from build123d import *

# Parameters (mm, degrees)
EXTRUDE001_DEPTH = 3
EXTRUDE_DEPTH    = 3
SKETCH_W         = 60
SKETCH_H         = 7
SKETCH_R         = 1.4
PAD_DEPTH        = 10
SKETCH001_W      = 60
SKETCH001_H      = 5
PAD001_DEPTH     = 3.5
SKETCH002_W      = 14
SKETCH002_H      = 5
PAD002_DEPTH     = 12
SKETCH003_R      = 1.9
PAD003_DEPTH     = 4


with BuildPart() as m2_5_pocket:
    # Polygon001 → Extrude001 (new body)
    with BuildSketch(Plane(origin=(56.6, 3, 10), x_dir=(1, 0, 0), z_dir=(0, 0, -1))):
        Polygon((1.45, 2.511474), (2.9, 0), (1.45, -2.511474), (-1.45, -2.511474), (-2.9, 0), (-1.45, 2.511474), align=None)
    extrude(amount=EXTRUDE001_DEPTH)


with BuildPart() as m2_5_pocket001:
    # Polygon → Extrude (new body)
    with BuildSketch(Plane(origin=(3.1, 3, 10), x_dir=(1, 0, 0), z_dir=(0, 0, -1))):
        Polygon((1.45, 2.511474), (2.9, 0), (1.45, -2.511474), (-1.45, -2.511474), (-2.9, 0), (-1.45, 2.511474), align=None)
    extrude(amount=EXTRUDE_DEPTH)


with BuildPart() as cut001:
    # Sketch → Pad (new body)
    with BuildSketch(Plane.XY):
        with Locations((30, 3.5)):
            Rectangle(SKETCH_W, SKETCH_H)
        with Locations((3.1, 3)):
            Circle(SKETCH_R, mode=Mode.SUBTRACT)
        with Locations((56.6, 3)):
            Circle(SKETCH_R, mode=Mode.SUBTRACT)
    extrude(amount=PAD_DEPTH)

    # Sketch001 → Pad001 (new body)
    with BuildSketch(Plane(origin=(0, 7, 0), x_dir=(-1, 0, 0), z_dir=(0, 1, 0))):
        with Locations((-30, 7.5)):
            Rectangle(SKETCH001_W, SKETCH001_H)
    extrude(amount=PAD001_DEPTH)

    # Sketch002 → Pad002 (new body)
    with BuildSketch(Plane(origin=(0, 7, 0), x_dir=(-1, 0, 0), z_dir=(0, 1, 0))):
        with Locations((-7, 7.5)):
            Rectangle(SKETCH002_W, SKETCH002_H)
    extrude(amount=PAD002_DEPTH)

    # Sketch003 → Pad003 (new body)
    with BuildSketch(Plane(origin=(0, 0, 5), x_dir=(1, 0, 0), z_dir=(0, 0, -1))):
        with Locations((7.3, -14.5)):
            Circle(SKETCH003_R)
    extrude(amount=PAD003_DEPTH)

    # Cut: cut M2.5 pocket001
    add(m2_5_pocket001.part, mode=Mode.SUBTRACT)

    # Cut001: cut M2.5 pocket
    add(m2_5_pocket.part, mode=Mode.SUBTRACT)


solid = cut001.part
Verification items for the finished model (mm, model axes). A direction names the side the tool comes from. Round coordinates to 2 decimals unless told otherwise and drop trailing zeros. Write each loop counter-clockwise with the first axis right and the second up, starting at its lowest first coordinate (ties: lowest second). Pieces come first, ordered by that corner, then holes.
(1) Depth check by flat-ended pin: pin 1 Ø2 at (y, z) = (13, 4.5) entering from +X; pin 2 Ø10 at (x, y) = (8, 12.5) entering from -Z; pin 3 Ø5.5 at (x, z) = (37.5, 8) entering from +Y; pin 4 Ø1.5 at (x, y) = (56.5, 2.5) entering from +Z. Enter the tip coordinate at first touch or a pass-through.
Returned:
pin 1: stops at x = 14
pin 2: stops at z = 1
pin 3: stops at y = 10.5
pin 4: passes through
(2) Section check C-C (z = 6.25). Enter the section's corners in (x, y).
Returned:
outline: (0, 0) - (60, 0) - (60, 10.5) - (14, 10.5) - (14, 19) - (0, 19) - close; hole circle Ø2.8 at (3.1, 3); hole circle Ø2.8 at (56.6, 3)
(3) Section check A-A (z = 2.5). Enter the section's corners in (x, y), plus the area to 3 significant figures.
Returned:
outline: (0, 0) - (60, 0) - (60, 7) - (0, 7) - close; circle Ø3.8 at (7.3, 14.5); hole circle Ø2.8 at (3.1, 3); hole circle Ø2.8 at (56.6, 3)
area: 419 mm2
(4) Mould release check, pull along X, two halves, no side actions. Record for faces 4 (the flat face through (30, 7, 2)), 5 (the flat face through (0, 7, 6)), 6 (the flat face through (58.785, 4.238, 8.521)): pulls with the +X half, pulls with the -X half, needs draft (parallel to the pull), parting line crosses it, or undercut.
Returned:
face 4: needs draft
face 5: pulls with the -X half
face 6: undercut
(5) Access from +Z, -Z, +X, -X, +Y, -Y to the whole of each face (thin tool, end or side, straight path). Record for faces 1 (the flat face through (0.935, 4.273, 8.521)), 2 (the cylindrical face through (5.4, 14.42, 3.03)), 3 (the flat face through (37, 10.5, 8)).
Returned:
face 1: +Z
face 2: -Z
face 3: +Z, -Z, +X, +Y
(6) Section check D-D (y = 3.75). Enter the section's corners in (x, z), plus the area to 3 significant figures.
Returned:
outline: (0, 0) - (1.92, 0) - (1.92, 7) - (0.63, 7) - (0.63, 10) - (0, 10) - close; (4.28, 0) - (55.42, 0) - (55.42, 7) - (54.13, 7) - (54.13, 10) - (5.57, 10) - (5.57, 7) - (4.28, 7) - close; (57.78, 0) - (60, 0) - (60, 10) - (59.07, 10) - (59.07, 7) - (57.78, 7) - close
area: 537 mm2
(7) Section check B-B (x = 56.6). Enter the section's corners in (y, z).
Returned:
outline: (0, 0) - (1.6, 0) - (1.6, 7) - (0.49, 7) - (0.49, 10) - (0, 10) - close; (4.4, 0) - (7, 0) - (7, 5) - (10.5, 5) - (10.5, 10) - (5.51, 10) - (5.51, 7) - (4.4, 7) - close
(8) Material ranges on line 1 (X direction, y = 3, z = 4.75); line 2 (Y direction, x = 3.1, z = 3); line 3 (X direction, y = 11.5, z = 8.5), recorded low to high.
Returned:
line 1: x = 0 to 1.7, 4.5 to 55.2, 58 to 60
line 2: y = 0 to 1.6, 4.4 to 7
line 3: x = 0 to 14
